```python
from build123d import *

# Parameters (mm, degrees)
BOSS_EXTRUDE1_DEPTH   = 100
SKETCH2_R             = 7.5
CUT_EXTRUDE1_DEPTH    = 525.690384894
FILLET1_R             = 10
BODY_MOVE_COPY1_ANGLE = 180


with BuildPart() as part:
    # Sketch1 → Boss-Extrude1 (new, symmetric)
    with BuildSketch(Plane.XY):
        with BuildLine():
            Line((440, -30), (-440, -30))
            ThreePointArc((-440, -30), (-470, 0), (-440, 30))
            Line((-440, 30), (110, 30))
            ThreePointArc((110, 30), (200, 120), (290, 30))
            Line((290, 30), (440, 30))
            Line((440, 30), (440, -30))
        make_face()
    extrude(amount=BOSS_EXTRUDE1_DEPTH, both=True)

    # Sketch2 → Cut-Extrude1 (cut, through all)
    with BuildSketch(Plane.XY.offset(100)):
        with Locations((-440, 0)):
            Circle(SKETCH2_R)
        with Locations((200, 80)):
            Circle(SKETCH2_R)
    extrude(amount=-CUT_EXTRUDE1_DEPTH, mode=Mode.SUBTRACT)

    # Fillet1
    fillet1_edges = [part.edges().sort_by_distance(p)[0] for p in [
        (110, 30, 0),
        (290, 30, 0),
    ]]
    fillet(fillet1_edges, radius=FILLET1_R)


with BuildPart() as part_1:
    # Body-Move/Copy1: moved
    add(part.part.rotate(Axis((0, 0, 0), (0, 0, 1)), BODY_MOVE_COPY1_ANGLE))


solid = part_1.part
```
Verification items for the finished model (mm, model axes). A direction names the side the tool comes from. Give positions to 0.01 mm unless a question says otherwise; leave off trailing zeros. Order: outer loops, then holes, each group sorted by start corner. A loop starts at its lowest first (then second) coordinate and runs counter-clockwise, first axis right, second up. Notation, with made-up numbers: (6.5, -21) - (35.5, -21) arc R8 ccw to (35.5, -15) - close; hole circle Ø1 at (60.25, 48). An arc over 180 degrees is marked (long way). Answer as CSV lines item,"result". Start each with the question number.
Item 1: Material ranges on L1, parallel to Y at x = 440, z = 37; L2, parallel to X at y = 0, z = 39.5; L3, parallel to Y at x = -200, z = 59.5, recorded low to high.
Item 2: Gauge pin test, flat ends, axial feed: pin 1 (2 mm diameter, centred on y = -38, z = -19.5, fed in from -X); pin 2 (12 mm diameter, centred on x = 440, y = 0, fed in from +Z); pin 3 (1.5 mm diameter, centred on y = -39.5, z = 71, fed in from +X); pin 4 (6 mm diameter, centred on y = 12.5, z = -23.5, fed in from +X). Record the tip position at first contact, or that the pin passes through.
Item 3: Section check C-C, the plane y = -104. Record the boundary of the cut face in (x, z) (3 decimals).
Item 4: Access from +Z, -Z, +X, -X, +Y, -Y to the whole of each face (thin tool, end or side, straight path). Record for faces 5 (the face through (-369, -30, 1)), 6 (the face through (9, -13, -100)).
Item 5: Section check A-A, the plane z = 72. Record the boundary of the cut face in (x, y), plus the area to 3 significant figures.
Item 6: Mould release check, pull along X, two halves, no side actions. Record for faces 1 (the face through (-440, 0, 1)), 2 (the face through (433.07, 2.87, 1.4)), 3 (the face through (469.993, 0.66, 1.4)), 4 (the face through (174, -30, 1)): released by +X, released by -X, zero draft, split by the parting line, or undercut.
Item 7: Section check B-B, the plane x = 44.5. Record the boundary of the cut face in (y, z).
Filled in:
1,L1,"-30 to -7.5, 7.5 to 30"
1,L2,"-440 to 432.5, 447.5 to 470"
1,L3,"-120 to -87.5, -72.5 to 30"
2,pin 1,"x = -289.96"
2,pin 2,"through"
2,pin 3,"x = -110.42"
2,pin 4,"x = 468.46"
3,outline,"(-251.225, -100) - (-148.775, -100) - (-148.775, 100) - (-251.225, 100) - close"
4,face 5,"+Z, -Z, -X, -Y"
4,face 6,"-Z, +X, -X, +Y, -Y"
5,outline,"(-440, -30) - (-299.5, -30) arc R10 cw to (-289.55, -39) arc R90 ccw to (-110.45, -39) arc R10 cw to (-100.5, -30) - (440, -30) arc R30 ccw to (440, 30) - (-440, 30) - close; hole circle Ø15 at (-200, -80); hole circle Ø15 at (440, 0)"
5,area,"66,600 mm^2"
6,face 1,"released by -X"
6,face 2,"undercut"
6,face 3,"released by +X"
6,face 4,"zero draft"
7,outline,"(-30, -100) - (30, -100) - (30, 100) - (-30, 100) - close"
